Design review of the part built by this model. Coordinates are the model's own, in mm. A direction names the side the tool comes from. Coordinates: 2 decimals unless noted, no trailing zeros. Write each loop counter-clockwise with the first axis right and the second up, starting at its lowest first coordinate (ties: lowest second). Pieces come first, ordered by that corner, then holes.
Q1. Take a section at B-B, the plane z = 0.75. Write out the cut boundary in (x, y), plus the area to 3 significant figures.
Q2. The part is to be moulded in two halves that separate along Y. For faces 4 (the flat face through (4, -5.3, 0)), 5 (the flat face through (3, -20.7, 0)), 6 (the flat face through (-0.52, -13, 0)), 7 (the flat face through (7.52, -13, 0)), say which applies: released by +Y, released by -Y, zero draft, split by the parting line, or undercut.
Q3. Take a section at C-C, the plane x = 2.25. Write out the cut boundary in (y, z).
Q4. For faces 1 (the flat face through (3.5, -5.8, 3.2)), 2 (the flat face through (3, -13, -3)), 3 (the flat face through (3, -13, 3)), list the 3-axis set-ups (+Z, -Z, +X, -X, +Y, -Y) from which the entire face can be reached by the end or side of a thin tool; tool diameter is ignored.
Q5. For pin 1 Ø4 at (y, z) = (-7, -2.5) entering from +X; pin 2 Ø2.5 at (x, y) = (2.5, -14) entering from -Z; pin 3 Ø4 at (y, z) = (-17, 2) entering from +X, all flat-tipped, find the tip position at first contact; note any pin that passes through.
Q6. Take a section at A-A, the plane x = 8. Write out the cut boundary in (y, z), plus the area to 3 significant figures.
Q7. For L1, parallel to Y at x = 8.25, z = -2; L2, parallel to X at y = -6, z = 1.75; L3, parallel to Z at x = 0.25, y = -8.5, list the stretches that pass through material, from the lowest coordinate up.
Q8. Take a section at D-D, the plane y = -7.5. Write out the cut boundary in (x, z), plus the area to 3 significant figures.
from build123d import *

# Parameters (mm, degrees)
SKETCH001_W  = 8.04
SKETCH001_H  = 14.4
PAD001_DEPTH = 3
SKETCH002_W  = 10
SKETCH002_H  = 7
PAD002_DEPTH = 0.5
SKETCH003_W  = 10
SKETCH003_H  = 7
PAD003_DEPTH = 0.5


with BuildPart() as part:
    # Sketch001 → Pad001 (new body, symmetric)
    with BuildSketch(Plane.XY):
        Rectangle(SKETCH001_W, SKETCH001_H)
    extrude(amount=PAD001_DEPTH, both=True)

    # Sketch002 (on Face3 of Pad001) → Pad002 (join)
    with BuildSketch(Plane.XZ.offset(7.2)):
        with Locations((0.02, 0)):
            Rectangle(SKETCH002_W, SKETCH002_H)
    extrude(amount=PAD002_DEPTH)

    # Sketch003 (on Face11 of Pad002) → Pad003 (join)
    with BuildSketch(Plane(origin=(0, 7.2, 0), x_dir=(-1, 0, 0), z_dir=(0, 1, 0))):
        with Locations((0.02, 0)):
            Rectangle(SKETCH003_W, SKETCH003_H)
    extrude(amount=PAD003_DEPTH)


with BuildPart() as part_1:
    # Body001 placement: moved
    add(part.part.moved(Location((3.5, -13, 0))))


solid = part_1.part
Responses:
1. outline: (-1.52, -5.8) - (-0.52, -5.8) - (-0.52, -20.2) - (-1.48, -20.2) - (-1.48, -20.7) - (8.52, -20.7) - (8.52, -20.2) - (7.52, -20.2) - (7.52, -5.8) - (8.48, -5.8) - (8.48, -5.3) - (-1.52, -5.3) - close
1. area: 126 mm2
2. face 4: released by +Y
2. face 5: released by -Y
2. face 6: undercut
2. face 7: undercut
3. outline: (-20.7, -3.5) - (-20.2, -3.5) - (-20.2, -3) - (-5.8, -3) - (-5.8, -3.5) - (-5.3, -3.5) - (-5.3, 3.5) - (-5.8, 3.5) - (-5.8, 3) - (-20.2, 3) - (-20.2, 3.5) - (-20.7, 3.5) - close
4. face 1: none
4. face 2: -Z, +X, -X
4. face 3: +Z, +X, -X
5. pin 1: stops at x = 8.48
5. pin 2: stops at z = -3
5. pin 3: stops at x = 7.52
6. outline: (-20.7, -3.5) - (-20.2, -3.5) - (-20.2, 3.5) - (-20.7, 3.5) - close; (-5.8, -3.5) - (-5.3, -3.5) - (-5.3, 3.5) - (-5.8, 3.5) - close
6. area: 7.00 mm2
7. L1: y = -20.7 to -20.2, -5.8 to -5.3
7. L2: x = -0.52 to 7.52
7. L3: z = -3 to 3
8. outline: (-0.52, -3) - (7.52, -3) - (7.52, 3) - (-0.52, 3) - close
8. area: 48.2 mm2
